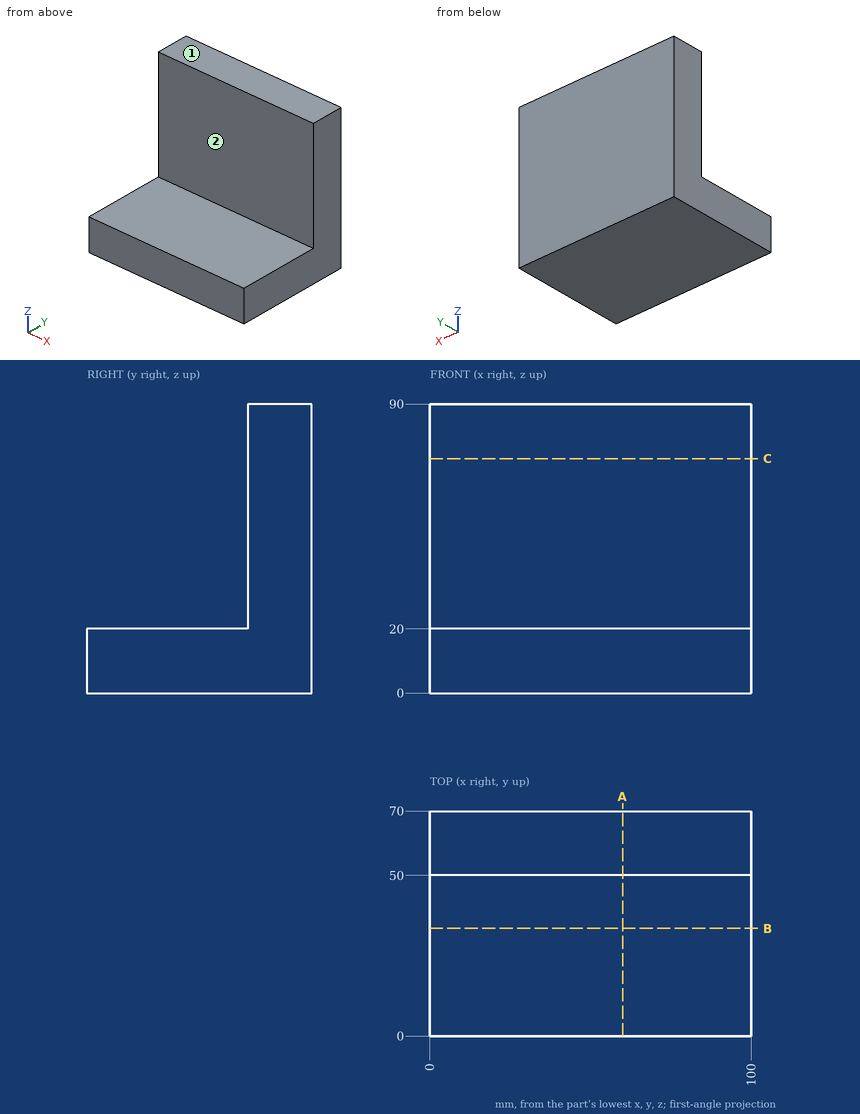
The drawing under review shows one solid part. Ordinate dimensions are in mm from its lowest x, y, z. A direction names the side the tool comes from. Coordinates: 2 decimals unless noted, no trailing zeros. Write each loop counter-clockwise with the first axis right and the second up, starting at its lowest first coordinate (ties: lowest second). Pieces come first, ordered by that corner, then holes. Notation, with made-up numbers: (23, -8.5) - (43, -8.5) arc R29 cw to (43, 22.5) - close; hole circle Ø10 at (62, 88). An arc over 180 degrees is marked (long way). Use one line per item in the form item = value.
Q1. For probe 1 along Z at (x, y) = (43, 42.5); probe 2 along Y at (x, z) = (44, 33.5), list the stretches that pass through material, from the lowest coordinate up.
Taken from the geometry:
probe_1 = 0 to 20
probe_2 = 50 to 70
Q2. Machinability: for the marked faces 1 and 2, which of the approach directions +Z, -Z, +X, -X, +Y, -Y give a long, thin tool a straight path to every point of the face, cutting with its end or side? Answer none if there is none.
Taken from the geometry:
face_1 = +Z, +X, -X, +Y, -Y
face_2 = +Z, +X, -X, -Y
Q3. Consider section B-B (y = 33.5). Write out the cut boundary in (x, z), plus the area to 3 significant figures.
Taken from the geometry:
outline = (0, 0) - (100, 0) - (100, 20) - (0, 20) - close
area = 2,000 mm^2
Q4. Consider section C-C (z = 73). Write out the cut boundary in (x, y).
Taken from the geometry:
outline = (0, 50) - (100, 50) - (100, 70) - (0, 70) - close
Q5. Consider section A-A (x = 60). Write out the cut boundary in (y, z), plus the area to 3 significant figures.
Taken from the geometry:
outline = (0, 0) - (70, 0) - (70, 90) - (50, 90) - (50, 20) - (0, 20) - close
area = 2,800 mm^2
Q6. Insertion check: pin 1 Ø3 at (x, y) = (64, 19) entering from +Z. The pin has a flat end and moves straight along its axis. Give the tip position at first contact, or say it passes through.
Taken from the geometry:
pin_1 = 20
